Here's the drawing with two shaded views (mm, measured from the low corner). I have some questions. Round coordinates to 2 decimals unless told otherwise and drop trailing zeros. Loops run counter-clockwise (first coordinate to the right, second up) from the corner with the lowest first, then second, coordinate; pieces in that order, holes last.
(1) I want a section at B-B on z = 18. Write out the boundary of the cut face in (x, y) (1 decimal).
(2) I want a section at A-A on x = 3.5. Write out the boundary of the cut face in (y, z).
(3) If I drill on line 1 along X through (y, z) = (3, 27.5) (1 decimal); line 2 along Z through (x, y) = (17, 3.7) (1 decimal); line 3 along X through (y, z) = (3.1, 3.5), over which ranges is the centre line in solid material (lowest first)?
(4) Thinking about a two-plate mould opening in X: for the marked faces 1, 2, 3 and 4, which applies, released by +X, released by -X, zero draft, split by the parting line, or undercut?
(5) Will these pins go through, and if not, where does the flat tip stop? pin 1 Ø2 at (x, z) = (17, 2) entering from -Y; pin 2 Ø2 at (y, z) = (1.5, 8) entering from +X; pin 3 Ø5 at (x, z) = (3.5, 27.5) entering from +Y; pin 4 Ø2 at (x, y) = (12, 1.5) entering from +Z.
(6) I want a section at D-D on z = 27.5. Write out the boundary of the cut face in (x, y), plus the area to 3 significant figures.
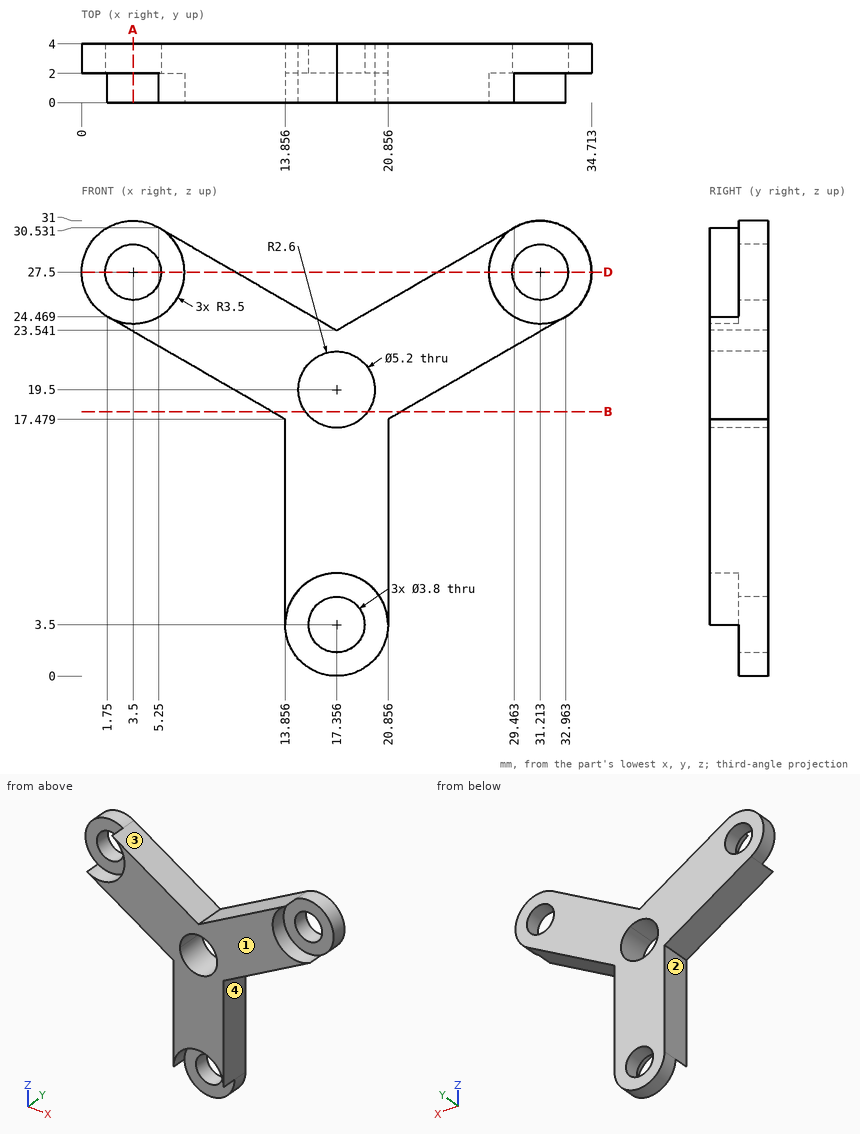
Filled sheet:
1. outline: (13, 0) - (15.2, 0) - (15.2, 4) - (13, 4) - close; (19.5, 0) - (21.8, 0) - (21.8, 4) - (19.5, 4) - close
2. outline: (0, 23.46) - (4, 23.46) - (4, 25.6) - (2, 25.6) - (2, 24) - (0, 24) - close; (2, 29.4) - (4, 29.4) - (4, 31) - (2, 31) - close
3. line 1: x = 0 to 1.6, 5.4 to 10.5, 24.2 to 29.3, 33.1 to 34.7
3. line 2: z = 0 to 1.6, 5.4 to 16.9, 22.1 to 23.7
3. line 3: x = 13.86 to 15.46, 19.26 to 20.86
4. face 1: zero draft
4. face 2: released by -X
4. face 3: undercut
4. face 4: released by +X
5. pin 1: stops at y = 2
5. pin 2: stops at x = 20.86
5. pin 3: stops at y = 4
5. pin 4: stops at z = 27.21
6. outline: (0, 2) - (1.6, 2) - (1.6, 4) - (0, 4) - close; (5.4, 2) - (7, 2) - (7, 0) - (10.5, 0) - (10.5, 4) - (5.4, 4) - close; (24.21, 0) - (27.71, 0) - (27.71, 2) - (29.31, 2) - (29.31, 4) - (24.21, 4) - close; (33.11, 2) - (34.71, 2) - (34.71, 4) - (33.11, 4) - close
6. area: 40.8 mm2
